Could you check a few things on this model? Use its own coordinates, in mm. Give positions to 0.01 mm unless a question says otherwise; leave off trailing zeros. Loops run counter-clockwise (first coordinate to the right, second up) from the corner with the lowest first, then second, coordinate; pieces in that order, holes last. Notation, with made-up numbers: M -25,-27.5 L 4,-27.5 A22 ccw 4,-10.5 Z; hole C 88,85.25 d4. An arc over 180 degrees is marked long. Return JSON: item names as keys, results as strings. Group by question number.
1. For pin 1 (1 mm diameter, centred on x = 10.5, y = -4.5, fed in from +Z), with a flat end and sliding along its axis, tell me the tip position at first contact or that it passes through.
2. If we section it at B-B (z = 1.5): Write out the boundary of the cut face in (x, y).
3. If we section it at A-A (y = 0): Write out the boundary of the cut face in (x, z).
4. Please list where these lines run through material, in increasing order: line 1 (X direction, y = -1, z = 1.4); line 2 (X direction, y = 5, z = 2); line 3 (X direction, y = 3, z = 1.55).
```python
from build123d import *

# Parameters (mm, degrees)
F0_R     = 2.5
F0_R_2   = 7.5
F1_DEPTH = 3
F2_R     = 1


with BuildPart() as f1:
    # F0 (on Top) → F1 (new body)
    with BuildSketch(Plane.XY):
        with BuildLine():
            ThreePointArc((34.8212002188, -15), (36.4142842854, 0), (34.8212002188, 15))
            Line((34.8212002188, 15), (-35, 10))
            Line((-35, 10), (-35, -10))
            Line((-35, -10), (34.8212002188, -15))
        make_face()
        Circle(F0_R, mode=Mode.SUBTRACT)
        with Locations((15, 0)):
            Circle(F0_R_2, mode=Mode.SUBTRACT)
    extrude(amount=F1_DEPTH)

    # F2
    f2_edges = [f1.edges().sort_by_distance(p)[0] for p in [
        (-35, 0, 3),
        (-0.0894, -12.5, 3),
        (36.414284, 0, 3),
        (-0.0894, 12.5, 3),
        (-2.5, 0, 3),
        (7.5, 0, 3),
    ]]
    fillet(f2_edges, radius=F2_R)


solid = f1.part
```
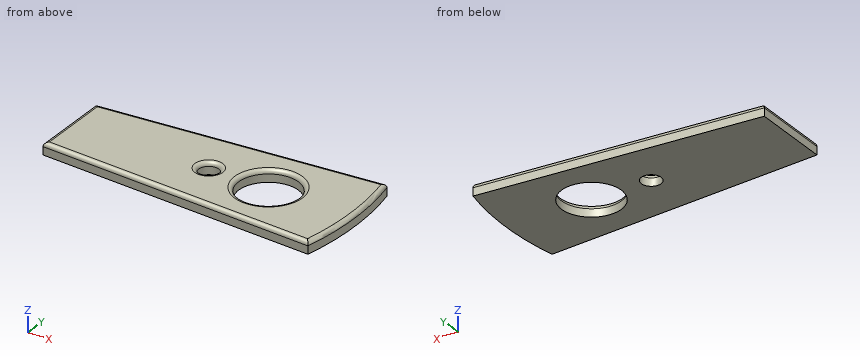
Answer:
{
 "1": {"pin 1": "passes through"},
 "2": {"outline": "M -35,-10 L 34.82,-15 A71.41 ccw 34.82,15 L -35,10 Z; hole C 0,0 d5; hole C 15,0 d15"},
 "3": {"outline": "M -35,0 L -2.5,0 L -2.5,2 A1 ccw -3.5,3 L -34,3 A1 ccw -35,2 Z; M 2.5,0 L 7.5,0 L 7.5,2 A1 ccw 6.5,3 L 3.5,3 A1 ccw 2.5,2 Z; M 22.5,0 L 36.41,0 L 36.41,2 A1 ccw 35.41,3 L 23.5,3 A1 ccw 22.5,2 Z"},
 "4": {"line 1": "x = -35 to -2.29, 2.29 to 7.57, 22.43 to 36.41", "line 2": "x = -35 to 9.41, 20.59 to 36.24", "line 3": "x = -35 to 8.13, 21.87 to 36.35"}
}
